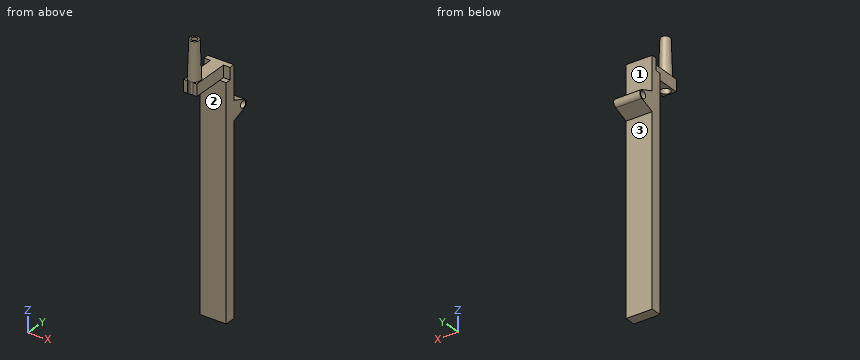
from build123d import *

# Parameters (mm, degrees)
BOSS_EXTRUDE2_DEPTH      = 27.94
BOSS_EXTRUDE2_DEPTH_BACK = 27.94
SKETCH3_R                = 7.62
SKETCH4_W                = 27.94
SKETCH4_H                = 25.4
BOSS_EXTRUDE3_DEPTH      = 80.01
CUT_EXTRUDE4_DEPTH       = 25.4
SKETCH9_R                = 9.9695
SKETCH10_R               = 12.7
SKETCH11_R               = 9.9695
SKETCH12_R               = 6.35
SKETCH14_W               = 55.88
SKETCH14_H               = 486.664
BOSS_EXTRUDE5_DEPTH      = 11.43


with BuildPart() as part:
    # Sketch3 → Boss-Extrude2 (new, two sides: drawn at the far end of the back side and taken through both)
    with BuildSketch(Plane(origin=(0, 0, 0), x_dir=(0, 0, -1), z_dir=(1, 0, 0)).offset(-BOSS_EXTRUDE2_DEPTH_BACK)):
        with BuildLine():
            Line((419.112, -27.6098), (28.956316714, -27.6098))
            Line((28.956316714, -27.6098), (20.9804, -27.6098))
            Line((20.9804, -27.6098), (8.875089173, 3.458094441))
            ThreePointArc((8.875089173, 3.458094441), (0, 9.525), (-8.875089173, 3.458094441))
            Line((-8.875089173, 3.458094441), (-20.9804, -27.6098))
            Line((-20.9804, -27.6098), (-28.958958547, -27.6098))
            Line((-28.958958547, -27.6098), (-92.952, -27.6098))
            Line((-92.952, -27.6098), (-92.952, -39.1795))
            Line((-92.952, -39.1795), (419.112, -39.1795))
            Line((419.112, -39.1795), (419.112, -27.6098))
        make_face()
        Circle(SKETCH3_R, mode=Mode.SUBTRACT)
    extrude(amount=BOSS_EXTRUDE2_DEPTH + BOSS_EXTRUDE2_DEPTH_BACK)

    # Sketch4 → Boss-Extrude3 (add)
    with BuildSketch(Plane.XZ.offset(39.1795)):
        with Locations((0, 80.252)):
            Rectangle(SKETCH4_W, SKETCH4_H)
    extrude(amount=BOSS_EXTRUDE3_DEPTH)

    # Sketch5 → Cut-Extrude4 (cut)
    with BuildSketch(Plane(origin=(0, 0, 67.552), x_dir=(-1, 0, 0), z_dir=(0, 0, -1))):
        with BuildLine():
            Line((6.02838635, -117.667539095), (6.02838635, -119.1895))
            Line((6.02838635, -119.1895), (0, -119.1895))
            ThreePointArc((0, -119.1895), (3.108770134, -118.803132618), (6.02838635, -117.667539095))
        make_face()
        with BuildLine():
            Line((0, -116.459), (0, -96.52))
            ThreePointArc((0, -96.52), (9.9695, -106.4895), (0, -116.459))
        make_face()
    cut_extrude4 = extrude(amount=-CUT_EXTRUDE4_DEPTH, mode=Mode.SUBTRACT)

    # Mirror1: Cut-Extrude4 across plane
    add(cut_extrude4.mirror(Plane(origin=(0, -116.459, 115.244479702), x_dir=(0, 0, 1), z_dir=(1, 0, 0))), mode=Mode.SUBTRACT)

    # Sketch9 → Loft1 section 0
    with BuildSketch(Plane.XY.offset(173.10039435)):
        with Locations((0, -106.4895)):
            Circle(SKETCH9_R)
    # Sketch10 → Loft1 section 1
    with BuildSketch(Plane.XY.offset(92.952)):
        with Locations((0, -106.4895)):
            Circle(SKETCH10_R)
    loft()

    # Sketch11 → Cut-Loft1 section 0
    with BuildSketch(Plane.XY.offset(92.952)):
        with Locations((0, -106.4895)):
            Circle(SKETCH11_R)
    # Sketch12 → Cut-Loft1 section 1
    with BuildSketch(Plane.XY.offset(173.10039435)):
        with Locations((0, -106.4895)):
            Circle(SKETCH12_R)
    loft(mode=Mode.SUBTRACT)

    # Sketch14 → Boss-Extrude5 (add)
    with BuildSketch(Plane.XZ.offset(39.1795)):
        with Locations((0, -175.78)):
            Rectangle(SKETCH14_W, SKETCH14_H)
    extrude(amount=BOSS_EXTRUDE5_DEPTH)


solid = part.part
Model file for the job. Use its own axes, mm. Face numbers are marked on the shaded views. A direction names the side the tool comes from. Coordinates: 2 decimals unless noted, no trailing zeros. Loops run counter-clockwise (first coordinate to the right, second up) from the corner with the lowest first, then second, coordinate; pieces in that order, holes last. Notation, with made-up numbers: (32, 69.25) -> (59, 69.25) arc R30 ccw to (59, 100.25) -> close; hole circle Ø5 at (-6, 87). An arc over 180 degrees is marked (long way). Use one line per item in the form item = value. Start each with the question number.
(1) Flat gauge pins, fed straight in: pin 1 (0.5 mm diameter, centred on y = -118.5, z = 76, fed in from +X); pin 2 (3 mm diameter, centred on x = -6, z = -123, fed in from -Y); pin 3 (5.5 mm diameter, centred on x = 21, y = -43.5, fed in from +Z); pin 4 (20 mm diameter, centred on y = 0, z = 0, fed in from +X). Where does each tip first touch, or does it go through?
(2) Cut at B-B on y = -82. Give the cut face in (x, z).
(3) Probe probe 1 along Y at (x, z) = (0, 76.5); probe 2 along Y at (x, z) = (-23.5, 85.5); probe 3 along Z at (x, y) = (-8.5, -92). List the from-to ranges inside material, lowest first. Write a range as from..to.
(4) Tool access for the marked faces 1, 2 and 3: list every direction of +Z, -Z, +X, -X, +Y, -Y with a clear straight run to the whole face (end or side of a thin tool).
(5) Cut at C-C on z = -350.5. Give the cut face in (x, y).
(6) Cut at A-A on z = 0. Give the cut face in (x, y) (1 decimal).
Values:
q1.pin_1 = 13.97
q1.pin_2 = -50.61
q1.pin_3 = 67.55
q1.pin_4 = 27.94
q2.outline = (-13.97, 67.55) -> (13.97, 67.55) -> (13.97, 92.95) -> (-13.97, 92.95) -> close
q3.probe_1 = -119.19..-116.46, -96.52..-27.61
q3.probe_2 = -39.18..-27.61
q3.probe_3 = 67.55..92.95
q4.face_1 = +Z, +X, -X, +Y
q4.face_2 = -Z, +X, -X, -Y
q4.face_3 = -Z, +X, -X, +Y
q5.outline = (-27.94, -50.61) -> (27.94, -50.61) -> (27.94, -27.61) -> (-27.94, -27.61) -> close
q6.outline = (-27.9, -50.6) -> (27.9, -50.6) -> (27.9, -7.6) -> (-27.9, -7.6) -> close; (-27.9, 7.6) -> (27.9, 7.6) -> (27.9, 9.5) -> (-27.9, 9.5) -> close
